Design review of the part shown in the three views and the two pictorial views. Dimensions are in mm from the part's minimum x, y and z. A direction names the side the tool comes from. Give positions to 0.01 mm unless a question says otherwise; leave off trailing zeros. Order: outer loops, then holes, each group sorted by start corner. A loop starts at its lowest first (then second) coordinate and runs counter-clockwise, first axis right, second up.
Item 1: Consider section B-B (y = 15.5). Give the boundary of the cut face in (x, z), plus the area to 3 significant figures.
Item 2: For P1, Ø8, axis at x = 58, y = 21.5, coming from the -Z side; P2, Ø6, axis at x = 70.5, z = 5, coming from the +Y side; P3, Ø3.5, axis at y = 14.5, z = 43, coming from the -X side, all flat-tipped, find the tip position at first contact; note any pin that passes through.
Item 3: Consider section C-C (z = 16). Give the boundary of the cut face in (x, y), plus the area to 3 significant figures.
Item 4: Machinability: for the marked faces 1, 2, 3 and 4, which of the approach directions +Z, -Z, +X, -X, +Y, -Y give a long, thin tool a straight path to every point of the face, cutting with its end or side? Answer none if there is none.
Item 5: Consider section D-D (x = 76.5). Give the boundary of the cut face in (y, z).
Item 6: For probe 1 along Z at (x, y) = (57.5, 16.5); probe 2 along X at (y, z) = (13.5, 9.5); probe 3 along Y at (x, z) = (14, 40), list the stretches that pass through material, from the lowest coordinate up.
Item 7: Consider section A-A (x = 54.5). Give the boundary of the cut face in (y, z).
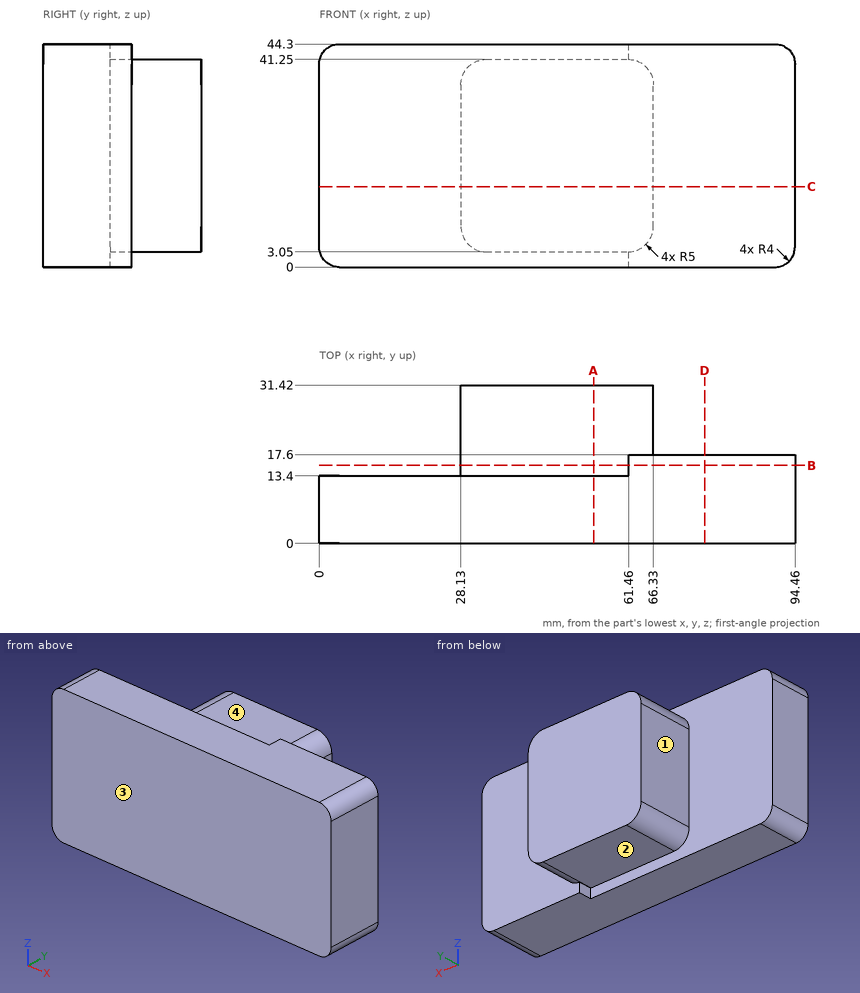
Resolved:
1. outline: (28.13, 8.05) arc R5 ccw to (33.13, 3.05) - (61.33, 3.05) arc R5 ccw to (61.46, 3.05) - (61.46, 0) - (90.46, 0) arc R4 ccw to (94.46, 4) - (94.46, 40.3) arc R4 ccw to (90.46, 44.3) - (61.46, 44.3) - (61.46, 41.25) arc R5 ccw to (61.33, 41.25) - (33.13, 41.25) arc R5 ccw to (28.13, 36.25) - close
1. area: 2,720 mm2
2. P1: stops at z = 3.05
2. P2: stops at y = 17.6
2. P3: stops at x = 0.23
3. outline: (0, 0) - (94.46, 0) - (94.46, 17.6) - (66.33, 17.6) - (66.33, 31.42) - (28.13, 31.42) - (28.13, 13.4) - (0, 13.4) - close
3. area: 2,070 mm2
4. face 1: +Z, -Z, -X, +Y
4. face 2: -Z, -X, +Y
4. face 3: +Z, -Z, +X, -X, -Y
4. face 4: +Z, -X, +Y
5. outline: (0, 0) - (17.6, 0) - (17.6, 44.3) - (0, 44.3) - close
6. probe 1: z = 3.05 to 41.25
6. probe 2: x = 28.13 to 94.46
6. probe 3: y = 0 to 13.4
7. outline: (0, 0) - (13.4, 0) - (13.4, 3.05) - (31.42, 3.05) - (31.42, 41.25) - (13.4, 41.25) - (13.4, 44.3) - (0, 44.3) - close
